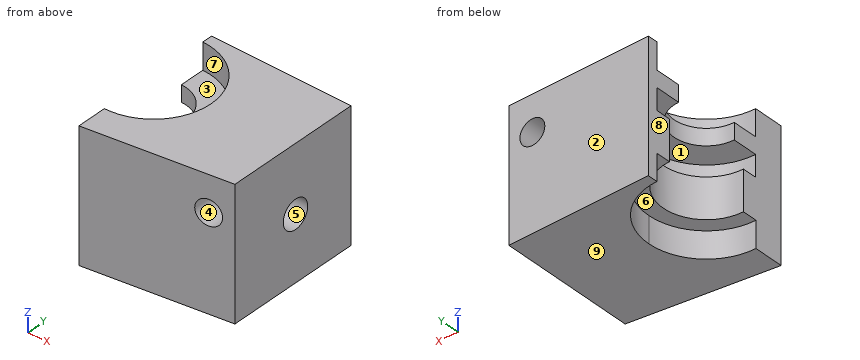
from build123d import *

# Parameters (mm, degrees)
F1_DEPTH       = 3.7
F3_DEPTH       = 5.6
F5_DEPTH       = 3
F7_DEPTH       = 2.3
F9_DEPTH       = 3.7
F11_DEPTH      = 25
F11_DEPTH_BACK = 25
F12_R          = 2
F13_DEPTH      = 7
F14_R          = 1.75
F15_DEPTH      = 25


with BuildPart() as f1:
    # F0 (on Top) → F1 (new body)
    with BuildSketch(Plane.XY):
        with BuildLine():
            Line((19.6, 9.5), (0, 12.21))
            Line((0, 12.21), (0, 8.1))
            ThreePointArc((0, 8.1), (5.7275649276, 5.7275649276), (8.1, 0))
            ThreePointArc((8.1, 0), (5.7275649276, -5.7275649276), (0, -8.1))
            Line((0, -8.1), (0, -12.21))
            Line((0, -12.21), (19.6, -9.5))
            Line((19.6, -9.5), (19.6, 0))
            Line((19.6, 0), (19.6, 9.5))
        make_face()
    extrude(amount=F1_DEPTH)

    # F2 (on face) → F3 (join)
    with BuildSketch(Plane.XY.offset(3.7)):
        with BuildLine():
            ThreePointArc((0, 6.05), (6.05, 0), (0, -6.05))
            Line((0, -6.05), (0, -8.1))
            Line((0, -8.1), (0, -12.21))
            Line((0, -12.21), (19.6, -9.5))
            Line((19.6, -9.5), (19.6, 9.5))
            Line((19.6, 9.5), (0, 12.21))
            Line((0, 12.21), (0, 8.1))
            Line((0, 8.1), (0, 6.05))
        make_face()
    extrude(amount=F3_DEPTH)

    # F4 (on face) → F5 (join)
    with BuildSketch(Plane.XY.offset(9.3)):
        with BuildLine():
            ThreePointArc((0, 8.05), (8.05, 0), (0, -8.05))
            Line((0, -8.05), (0, -12.21))
            Line((0, -12.21), (19.6, -9.5))
            Line((19.6, -9.5), (19.6, 9.5))
            Line((19.6, 9.5), (0, 12.21))
            Line((0, 12.21), (0, 8.05))
        make_face()
    extrude(amount=F5_DEPTH)

    # F6 (on face) → F7 (join)
    with BuildSketch(Plane.XY.offset(12.3)):
        with BuildLine():
            ThreePointArc((0, 4.55), (4.55, 0), (0, -4.55))
            Line((0, -4.55), (0, -12.21))
            Line((0, -12.21), (19.6, -9.5))
            Line((19.6, -9.5), (19.6, 9.5))
            Line((19.6, 9.5), (0, 12.21))
            Line((0, 12.21), (0, 4.55))
        make_face()
    extrude(amount=F7_DEPTH)

    # F8 (on face) → F9 (join)
    with BuildSketch(Plane.XY.offset(14.6)):
        with BuildLine():
            ThreePointArc((0, 8.05), (8.05, 0), (0, -8.05))
            Line((0, -8.05), (0, -12.21))
            Line((0, -12.21), (19.6, -9.5))
            Line((19.6, -9.5), (19.6, 9.5))
            Line((19.6, 9.5), (0, 12.21))
            Line((0, 12.21), (0, 8.05))
        make_face()
    extrude(amount=F9_DEPTH)

    # F10 (on face) → F11 (cut, two sides)
    with BuildSketch(Plane(origin=(0, 0, 0), x_dir=(1, 0, 0), z_dir=(0, 0, -1))) as f11_sk:
        Polygon((0, -12.21), (19.6, -9.5), (0, -9.5), align=None)
    extrude(amount=-F11_DEPTH, mode=Mode.SUBTRACT)
    extrude(f11_sk.sketch, amount=F11_DEPTH_BACK, mode=Mode.SUBTRACT)

    # F12 (on face) → F13 (cut)
    with BuildSketch(Plane.YZ.offset(19.6)):
        with Locations((0.4, 9)):
            Circle(F12_R)
    extrude(amount=-F13_DEPTH, mode=Mode.SUBTRACT)

    # F14 (on face) → F15 (cut)
    with BuildSketch(Plane(origin=(0, 9.5, 0), x_dir=(-1, 0, 0), z_dir=(0, 1, 0))):
        with Locations((-16.3, 13.3)):
            Circle(F14_R)
    extrude(amount=-F15_DEPTH, mode=Mode.SUBTRACT)


solid = f1.part
The model under review builds one solid part; all positions refer to its coordinate system, in mm. Face numbers are marked on the shaded views. A direction names the side the tool comes from. Coordinates: 2 decimals unless noted, no trailing zeros. Write each loop counter-clockwise with the first axis right and the second up, starting at its lowest first coordinate (ties: lowest second). Pieces come first, ordered by that corner, then holes. Notation, with made-up numbers: (-25, 79) - (-8, 79) arc R27 ccw to (-8, 117) - close; hole circle Ø10 at (20.25, 49.5). An arc over 180 degrees is marked (long way). Answer as CSV lines item,"result".
(1) We need section A-A (x = 16.5). Give the boundary of the cut face in (y, z).
Data:
outline,"(-9.93, 0) - (9.5, 0) - (9.5, 11.56) - (-9.93, 11.56) - close; (-9.93, 15.04) - (9.5, 15.04) - (9.5, 18.3) - (-9.93, 18.3) - close; hole circle Ø4 at (0.4, 9)"
(2) For line 1 along Z through (x, y) = (15.5, 0.4); line 2 along Z through (x, y) = (14.5, 0.4); line 3 along Z through (x, y) = (16.3, 2.5), list the stretches that pass through material, from the lowest coordinate up. Write a range as [from, to].
Data:
line 1,"z = [0, 7], [11, 11.74], [14.86, 18.3]"
line 2,"z = [0, 7], [11, 18.3]"
line 3,"z = [0, 11.55], [15.05, 18.3]"
(3) We need section C-C (y = -4). Give the boundary of the cut face in (x, z).
Data:
outline,"(2.17, 12.3) - (6.99, 12.3) - (6.99, 9.3) - (4.54, 9.3) - (4.54, 3.7) - (7.04, 3.7) - (7.04, 0) - (19.6, 0) - (19.6, 18.3) - (6.99, 18.3) - (6.99, 14.6) - (2.17, 14.6) - close; hole circle Ø3.5 at (16.3, 13.3)"
(4) Mouldability with a two-part tool opening along Y and no side actions: class the marked faces 1, 2, 3 and 4 as pulls with the +Y half, pulls with the -Y half, needs draft (parallel to the pull), parting line crosses it, or undercut.
Data:
face 1,"undercut"
face 2,"pulls with the +Y half"
face 3,"undercut"
face 4,"needs draft"
(5) We need section B-B (z = 1.5). Give the boundary of the cut face in (x, y), plus the area to 3 significant figures.
Data:
outline,"(0, -12.21) - (19.6, -9.5) - (19.6, 9.5) - (0, 9.5) - (0, 8.1) arc R8.1 cw to (0, -8.1) - close"
area,"296 mm2"
(6) Tool access review of the marked faces 5, 6, 7, 8 and 9: name each direction out of +Z, -Z, +X, -X, +Y, -Y from which nothing blocks a thin tool from reaching the whole face with its end or side.
Data:
face 5,"+X"
face 6,"-Z, -X"
face 7,"+Z, -X"
face 8,"+Z, -Z, -X, +Y, -Y"
face 9,"-Z, +X, -X, +Y, -Y"
(7) Clearance check with flat-ended pins moving along their axes: pin 1 Ø4 at (x, z) = (16.3, 13.3) entering from -Y; pin 2 Ø2.5 at (x, y) = (3.5, -3) entering from -Z; pin 3 Ø2 at (y, z) = (0, 4) entering from -X. State where each tip first meets the part, or that it passes through.
Data:
pin 1,"stops at y = -10.23"
pin 2,"stops at z = 12.3"
pin 3,"stops at x = 5.97"
(8) We need section D-D (z = 13.3). Give the boundary of the cut face in (x, y).
Data:
outline,"(0, -12.21) - (14.55, -10.2) - (14.55, 9.5) - (0, 9.5) - (0, 4.55) arc R4.55 cw to (0, -4.55) - close; (18.05, -9.71) - (19.6, -9.5) - (19.6, 9.5) - (18.05, 9.5) - close"
